from build123d import *

# Parameters (mm, degrees)
ESBO_O1_R                = 9.5
RESSALTO_EXTRUS_O1_DEPTH = 25
ESBO_O2_R                = 4
CORTE_EXTRUS_O1_DEPTH    = 12.5
ESBO_O3_R                = 2.5
CORTE_EXTRUS_O2_DEPTH    = 26
ESBO_O4_R                = 1.5
CORTE_EXTRUS_O3_DEPTH    = 12
ESBO_O5_R                = 1.5
CORTE_EXTRUS_O4_DEPTH    = 10.5000001


with BuildPart() as part:
    # Esboço1 → Ressalto-extrusão1 (new body)
    with BuildSketch(Plane.XY):
        Circle(ESBO_O1_R)
    extrude(amount=RESSALTO_EXTRUS_O1_DEPTH)

    # Esboço2 → Corte-extrusão1 (cut)
    with BuildSketch(Plane.XY.offset(25)):
        Circle(ESBO_O2_R)
    extrude(amount=-CORTE_EXTRUS_O1_DEPTH, mode=Mode.SUBTRACT)

    # Esboço3 → Corte-extrusão2 (cut, through all)
    with BuildSketch(Plane(origin=(0, 0, 0), x_dir=(-1, 0, 0), z_dir=(0, 0, -1))):
        Circle(ESBO_O3_R)
    extrude(amount=-CORTE_EXTRUS_O2_DEPTH, mode=Mode.SUBTRACT)

    # Esboço4 → Corte-extrusão3 (cut)
    with BuildSketch(Plane(origin=(0, 0, 0), x_dir=(1, 0, 0), z_dir=(0, 1, 0))):
        with Locations((0, -4)):
            Circle(ESBO_O4_R)
        with Locations((0, -21)):
            Circle(ESBO_O4_R)
    extrude(amount=CORTE_EXTRUS_O3_DEPTH, mode=Mode.SUBTRACT)

    # Esboço5 → Corte-extrusão4 (cut, through all)
    with BuildSketch(Plane(origin=(0, 0, 0), x_dir=(0, 0, -1), z_dir=(1, 0, 0))):
        with Locations((-21, 0)):
            Circle(ESBO_O5_R)
        with Locations((-4, 0)):
            Circle(ESBO_O5_R)
    extrude(amount=-CORTE_EXTRUS_O4_DEPTH, mode=Mode.SUBTRACT)


solid = part.part
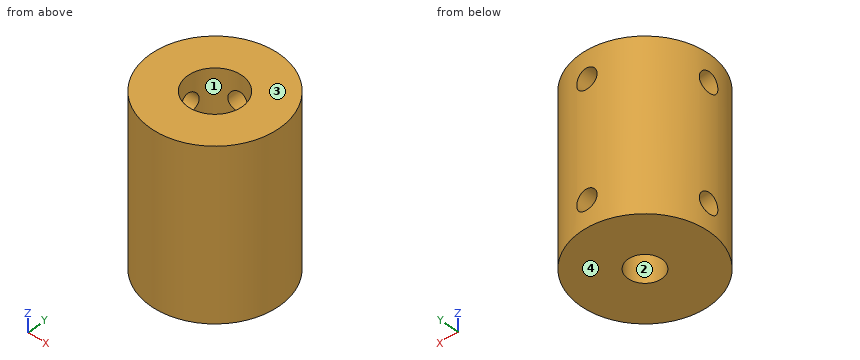
Source: CAD feature listing. Evaluate the final solid. Frame: model axes, mm. Face numbers are marked on the shaded views. A direction names the side the tool comes from. Round coordinates to 2 decimals unless told otherwise and drop trailing zeros. Loops run counter-clockwise (first coordinate to the right, second up) from the corner with the lowest first, then second, coordinate; pieces in that order, holes last. Notation, with made-up numbers: M -15,53 L 40,53 A24 ccw 40,65 Z; hole C 16,-9 d2. An arc over 180 degrees is marked long. Return JSON: item names as keys, results as strings. Group by question number.
1. Material intervals for line 1 along X through (y, z) = (0, 22.75); line 2 along X through (y, z) = (6.6, 21); line 3 along Z through (x, y) = (-0.5, 8.5), sorted ascending. Write a range as from..to.
2. Section query A-A on y = 0. Output: boundary loops of the cut face in (x, z).
3. Section query B-B on z = 21. Output: boundary loops of the cut face in (x, y), and give its area (3 significant figures).
4. Section query C-C on x = 0. Output: boundary loops of the cut face in (y, z), and give its area (3 significant figures).
5. Mould query, pull axis Z, two halves, no side actions, for the marked faces 3 and 4. Classes: released by +Z, released by -Z, zero draft, split by the parting line, or undercut.
6. Reachability of the marked faces 1 and 2 from +Z, -Z, +X, -X, +Y, -Y: full face, straight path, thin tool, end or side. Return the list, or none.
7. Section query D-D on x = -3.25. Output: boundary loops of the cut face in (y, z).
8. Pin query (flat end, axial travel): pin 1 (1 mm diameter, centred on y = -7.5, z = 5, fed in from -X); pin 2 (6 mm diameter, centred on y = 4, z = 16.5, fed in from -X); pin 3 (8 mm diameter, centred on y = 5.5, z = 22, fed in from +X). Return the tip coordinate at first contact, or that it passes through.
Checks:
{
 "1": {"line 1": "x = -9.5..-4, 4..9.5", "line 2": "x = -6.83..-1.5, 1.5..6.83", "line 3": "z = 0..2.59, 5.41..19.59, 22.41..25"},
 "2": {"outline": "M -9.5,0 L -2.5,0 L -2.5,2.5 L -9.5,2.5 Z; M -9.5,5.5 L -2.5,5.5 L -2.5,12.5 L -4,12.5 L -4,19.5 L -9.5,19.5 Z; M -9.5,22.5 L -4,22.5 L -4,25 L -9.5,25 Z; M 2.5,0 L 9.5,0 L 9.5,25 L 4,25 L 4,12.5 L 2.5,12.5 Z"},
 "3": {"outline": "M -9.38,-1.5 A9.5 ccw long 1.5,9.38 L 1.5,3.71 A4 cw long -3.71,-1.5 Z; M -9.38,1.5 L -3.71,1.5 A4 cw -1.5,3.71 L -1.5,9.38 A9.5 ccw Z", "area": "200 mm²"},
 "4": {"outline": "M -9.5,0 L -2.5,0 L -2.5,12.5 L -4,12.5 L -4,25 L -9.5,25 Z; M 2.5,0 L 9.5,0 L 9.5,2.5 L 2.5,2.5 Z; M 2.5,5.5 L 9.5,5.5 L 9.5,19.5 L 4,19.5 L 4,12.5 L 2.5,12.5 Z; M 4,22.5 L 9.5,22.5 L 9.5,25 L 4,25 Z", "area": "275 mm²"},
 "5": {"face 3": "released by +Z", "face 4": "released by -Z"},
 "6": {"face 1": "+Z", "face 2": "+Z, -Z"},
 "7": {"outline": "M -8.93,0 L 8.93,0 L 8.93,25 L 2.33,25 L 2.33,12.5 L -2.33,12.5 L -2.33,25 L -8.93,25 Z; hole C 0,4 d3"},
 "8": {"pin 1": "stops at x = -6.42", "pin 2": "stops at x = -9.45", "pin 3": "stops at x = 9.38"}
}
